```python
from build123d import *

# Parameters (mm, degrees)
F1_DEPTH = 6.35
F2_R     = 2.35839
F3_DEPTH = 6.351


with BuildPart() as f1:
    # F0 (on Right) → F1 (new body)
    with BuildSketch(Plane.YZ):
        Polygon((-196.85, 38.1), (-196.85, 0), (196.85, 0), (196.85, 127), (-107.95, 127), align=None)
    extrude(amount=F1_DEPTH)

    # F2 (on face) → F3 (cut, through all)
    with BuildSketch(Plane.YZ.offset(6.35)):
        with Locations((53.975, 57.15)):
            Circle(F2_R)
        with Locations((63.5, 57.15)):
            Circle(F2_R)
        with Locations((73.025, 57.15)):
            Circle(F2_R)
    extrude(amount=-F3_DEPTH, mode=Mode.SUBTRACT)


solid = f1.part
```
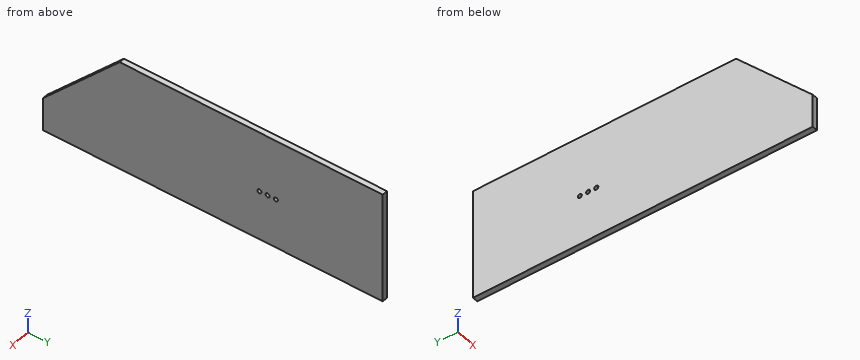
Geometry check sheet. Reference: the model listing, model coordinates, mm. Round coordinates to 2 decimals unless told otherwise and drop trailing zeros. Loops run counter-clockwise (first coordinate to the right, second up) from the corner with the lowest first, then second, coordinate; pieces in that order, holes last. Notation, with made-up numbers: (4.5, 76) - (24.5, 76) arc R17 ccw to (24.5, 103) - close; hole circle Ø5 at (-11, 10.5). An arc over 180 degrees is marked (long way). Write each question's results on one line, items separated by ' | '. Start each with the question number.
Q1. Cross-section at A-A on x = 4.25. Enter the section's corners in (y, z) (3 decimals), and give its area (3 significant figures).
Q2. Thickness scan on line 1 (Z direction, x = 3.5, y = 63.5); line 2 (Z direction, x = 4.25, y = 53); line 3 (Y direction, x = 3.5, z = 110). Record the ranges inside material, lowest first. Write a range as [from, to].
Q3. Cross-section at B-B on z = 78.5. Enter the section's corners in (x, y), and give its area (3 significant figures).
Answers below:
1) outline: (-196.85, 0) - (196.85, 0) - (196.85, 127) - (-107.95, 127) - (-196.85, 38.1) - close; hole circle Ø4.717 at (53.975, 57.15); hole circle Ø4.717 at (63.5, 57.15); hole circle Ø4.717 at (73.025, 57.15) | area: 46,000 mm²
2) line 1: z = [0, 54.79], [59.51, 127] | line 2: z = [0, 55], [59.3, 127] | line 3: y = [-124.95, 196.85]
3) outline: (0, -156.45) - (6.35, -156.45) - (6.35, 196.85) - (0, 196.85) - close | area: 2,240 mm²
